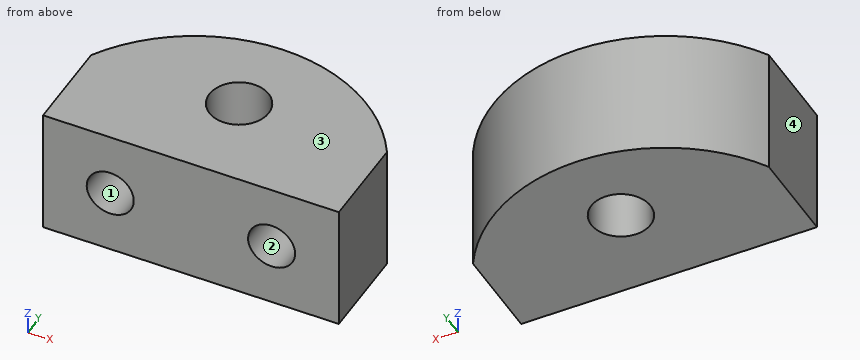
```python
from build123d import *

# Parameters (mm, degrees)
EXTRUDE_3_8_DEPTH = 9.63
SKETCH2_R         = 2.2
M5_DRILL_DEPTH    = 9.63
SKETCH3_R         = 1.75
M4_DRILL_DEPTH    = 8


with BuildPart() as part:
    # Sketch1 → 3/8 (new body)
    with BuildSketch(Plane.XY):
        with BuildLine():
            Line((-11, 3.5), (-11, -3.5))
            Line((-11, -3.5), (11, -3.5))
            Line((11, -3.5), (11, 3.5))
            ThreePointArc((11, 3.5), (0, 9.776932339), (-11, 3.5))
        make_face()
    extrude(amount=EXTRUDE_3_8_DEPTH)

    # Sketch2 → M5_DRILL (cut)
    with BuildSketch(Plane.XY.offset(9.63)):
        with Locations((0, 3.5)):
            Circle(SKETCH2_R)
    extrude(amount=-M5_DRILL_DEPTH, mode=Mode.SUBTRACT)

    # Sketch3 → M4_DRILL (cut)
    with BuildSketch(Plane.XZ.offset(3.5)):
        with Locations(Location((-6, 4.815, 0), (0, 0, 270))):
            Circle(SKETCH3_R)
        with Locations(Location((6, 4.815, 0), (0, 0, 90))):
            Circle(SKETCH3_R)
    extrude(amount=-M4_DRILL_DEPTH, mode=Mode.SUBTRACT)


solid = part.part
```
For this review, take the finished solid that the model builds, in its own axes (mm). Face numbers are marked on the shaded views. Round coordinates to 2 decimals unless told otherwise and drop trailing zeros. Write each loop counter-clockwise with the first axis right and the second up, starting at its lowest first coordinate (ties: lowest second). Pieces come first, ordered by that corner, then holes. Notation, with made-up numbers: (-19.75, -35) - (-0.75, -35) arc R5 ccw to (-0.75, -26) - close; hole circle Ø5 at (-32, 3). An arc over 180 degrees is marked (long way). Answer as CSV lines item,"result". Start each with the question number.
(1) For pin 1 (1 mm diameter, centred on y = 5, z = 7.5, fed in from -X); pin 2 (1 mm diameter, centred on x = -6, z = 5, fed in from -Y); pin 3 (3 mm diameter, centred on x = -6, z = 4.815, fed in from +Y), all flat-tipped, find the tip position at first contact; note any pin that passes through.
(2) Mouldability with a two-part tool opening along Z and no side actions: class the marked faces 1, 2, 3 and 4 as +Z half, -Z half, draft (parallel to the pull), parting line (faces both ways), or undercut.
(3) Add section D-D, the plane x = 6. State the section outline as (y, z) points (3 decimals), plus the area to 3 significant figures.
(4) Add section B-B, the plane z = 8.75. State the section outline as (x, y) points.
(5) For line 1 (X direction, y = 4.25, z = 4); line 2 (Y direction, x = 1.5, z = 5); line 3 (Y direction, x = -0.5, z = 6), list the stretches that pass through material, from the lowest coordinate up.
(6) Add section C-C, the plane y = -0.5. State the section outline as (x, z) points (3 decimals).
(7) Add section A-A, the plane x = 0.5. State the section outline as (y, z) points.
From the geometry:
1,pin 1,"stops at x = -10.34"
1,pin 2,"stops at y = 4.5"
1,pin 3,"stops at y = 8.96"
2,face 1,"undercut"
2,face 2,"undercut"
2,face 3,"+Z half"
2,face 4,"draft"
3,outline,"(-3.5, 0) - (8.281, 0) - (8.281, 9.63) - (-3.5, 9.63) - (-3.5, 6.565) - (4.5, 6.565) - (4.5, 3.065) - (-3.5, 3.065) - close"
3,area,"85.4 mm²"
4,outline,"(-11, -3.5) - (11, -3.5) - (11, 3.5) arc R12.78 ccw to (-11, 3.5) - close; hole circle Ø4.4 at (0, 3.5)"
5,line 1,"x = -10.52 to -7.55, -4.45 to -2.07, 2.07 to 4.45, 7.55 to 10.52"
5,line 2,"y = -3.5 to 1.89, 5.11 to 9.69"
5,line 3,"y = -3.5 to 1.36, 5.64 to 9.77"
6,outline,"(-11, 0) - (11, 0) - (11, 9.63) - (-11, 9.63) - close; hole circle Ø3.5 at (-6, 4.815); hole circle Ø3.5 at (6, 4.815)"
7,outline,"(-3.5, 0) - (1.36, 0) - (1.36, 9.63) - (-3.5, 9.63) - close; (5.64, 0) - (9.77, 0) - (9.77, 9.63) - (5.64, 9.63) - close"
